Solid Edge part; units mm, degrees
sketch "Sketch1" plane through (0, 0, 0) normal (0, 0, 1) x (1, 0, 0)
  circle A0 centre (15, 15) radius 1.7
  line L0 (-5, -60) -> (20, -60)
  line L1 (20, -60) -> (20, 20)
  line L2 (20, 20) -> (-5, 20)
  line L3 (-5, 20) -> (-5, -60)
  circle A1 centre (0, 0) radius 1.7
  dimension "D1" = 15
  dimension "D2" = 5
extrude "Protrusion1" add sketch "Sketch1" along normal blind 5
properties material "Steel"
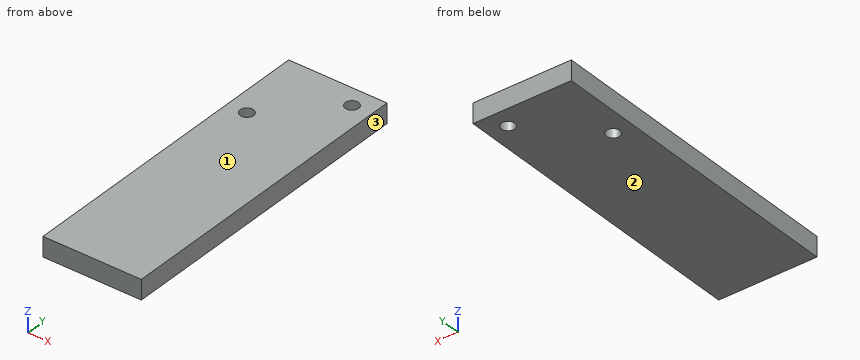
CAD build for the part. Positions are in the model's coordinates, mm. Face numbers are marked on the shaded views. Give positions to 0.01 mm unless a question says otherwise; leave off trailing zeros. Order: outer loops, then holes, each group sorted by start corner. A loop starts at its lowest first (then second) coordinate and runs counter-clockwise, first axis right, second up.
(1) Mould opens along Z. For the marked faces 1, 2 and 3 say: released by +Z, released by -Z, zero draft, split by the parting line, or undercut.
(2) Saw through at A-A, the plane y = 15. Give the cut face in (x, z).
(3) Drill centre lines: L1, parallel to Y at x = 15, z = 1.7; L2, parallel to Y at x = 0, z = 2.8. Where is each one in solid material? Low to high.
(4) Saw through at B-B, the plane x = 15. Give the cut face in (y, z).
Results found:
1. face 1: released by +Z
1. face 2: released by -Z
1. face 3: zero draft
2. outline: (-5, 0) - (13.3, 0) - (13.3, 5) - (-5, 5) - close; (16.7, 0) - (20, 0) - (20, 5) - (16.7, 5) - close
3. L1: y = -60 to 13.3, 16.7 to 20
3. L2: y = -60 to -1.7, 1.7 to 20
4. outline: (-60, 0) - (13.3, 0) - (13.3, 5) - (-60, 5) - close; (16.7, 0) - (20, 0) - (20, 5) - (16.7, 5) - close
